Build history of the part. All positions in model axes, mm. A direction names the side the tool comes from. Give positions to 0.01 mm unless a question says otherwise; leave off trailing zeros. Write each loop counter-clockwise with the first axis right and the second up, starting at its lowest first coordinate (ties: lowest second). Pieces come first, ordered by that corner, then holes. Notation, with made-up numbers: (18, 35) -> (26, 35) arc R29 cw to (26, 55) -> close; hole circle Ø7 at (27, 81.5). An arc over 180 degrees is marked (long way). Put each result on its own line as item: value. Start each with the question number.
Item 1: Slice it at A-A, the plane x = 45.04. List the corners of the cut face in (y, z).
Item 2: Slice it at C-C, the plane z = -6.5. Give the number of separate pieces and of enclosed holes in the cut face, plus the area to 3 significant figures.
Item 3: Tool access for faces 4 (the flat face through (39, -45, -1.8)), 5 (the flat face through (39, -45, -8.3)), 6 (the flat face through (47.15, -32, -5)): list every direction of +Z, -Z, +X, -X, +Y, -Y with a clear straight run to the whole face (end or side of a thin tool).
Item 4: Flat gauge pins, fed straight in: pin 1 Ø4 at (x, z) = (39.5, -4.5) entering from -Y; pin 2 Ø3 at (x, z) = (48, -5.5) entering from +Y; pin 3 Ø1.3 at (y, z) = (-69, -5) entering from -X; pin 4 Ø1.5 at (y, z) = (-54.5, -1.5) entering from +X. Where does each tip first touch, or does it go through?
Item 5: Slice it at D-D, the plane x = 40. List the corners of the cut face in (y, z), plus the area to 3 significant figures.
Item 6: Slice it at B-B, the plane y = -31.5. List the corners of the cut face in (x, z), plus the area to 3 significant figures.
Item 7: Drill centre lines: line 1 along X through (y, z) = (-39.04, -4.25); line 2 along X through (y, z) = (-33, -6.75); line 3 along Y through (x, z) = (50.25, -6.5). Where is each one in solid material? Low to high.
Item 8: Two-plate mould, pull along X, no slides. Class faces 1 (the flat face through (52.05, -32, -5)), 2 (the flat face through (60.34, -60.4, -5.02)), 3 (the flat face through (60, -64, -2.925)): pulls with the +X half, pulls with the -X half, needs draft (parallel to the pull), parting line crosses it, or undercut.
```python
from build123d import *

# Parameters (mm, degrees)
SKETCH037_W             = 27.9
SKETCH037_H             = 15.9
SKETCH037_R             = 1.75
PAD025_DEPTH            = 9.9
SKETCH038_W             = 27.7
SKETCH038_H             = 4.25
REVOLUTION_ANGLE        = 10
SKETCH039_W             = 0.8
SKETCH039_H             = 6.5
PAD026_DEPTH            = 8.9
SKETCH040_W             = 0.8
SKETCH040_H             = 6.5
PAD027_DEPTH            = 3.5
SKETCH041_W             = 0.8
SKETCH041_H             = 6.5
PAD028_DEPTH            = 8.9
BODY007_PLACEMENT_ANGLE = 90


with BuildPart() as obj1:
    # Sketch037 → Pad025 (new body)
    with BuildSketch(Plane.XY):
        Rectangle(SKETCH037_W, SKETCH037_H)
        with Locations((10.96, 4.96)):
            Circle(SKETCH037_R, mode=Mode.SUBTRACT)
        with Locations((-10.96, -4.96)):
            Circle(SKETCH037_R, mode=Mode.SUBTRACT)
    extrude(amount=PAD025_DEPTH)

    # Sketch038 (on Face3 of Pad025) → Revolution (revolve)
    with BuildSketch(Plane.XZ.offset(7.95)):
        with Locations((10.8, 4.95)):
            Rectangle(SKETCH038_W, SKETCH038_H)
    revolve(axis=Axis((-3.15, -7.95, 7.075), (0, 0, -1)), revolution_arc=REVOLUTION_ANGLE)

    # Sketch039 (on Face2 of Revolution) → Pad026 (join)
    with BuildSketch(Plane(origin=(-13.95, 0, 0), x_dir=(0, -1, 0), z_dir=(-1, 0, 0))):
        with Locations((-2.45, 4.95)):
            Rectangle(SKETCH039_W, SKETCH039_H)
        with Locations((2.45, 4.95)):
            Rectangle(SKETCH039_W, SKETCH039_H)
    extrude(amount=PAD026_DEPTH)

    # Sketch040 (on Face1 of Pad026) → Pad027 (join)
    with BuildSketch(Plane(origin=(0, 7.95, 0), x_dir=(-1, 0, 0), z_dir=(0, 1, 0))):
        with Locations((1.55, 4.95)):
            Rectangle(SKETCH040_W, SKETCH040_H)
    extrude(amount=PAD027_DEPTH)

    # Sketch041 (on Face8 of Pad027) → Pad028 (join)
    with BuildSketch(Plane(origin=(-1.95, 0, 0), x_dir=(0, -1, 0), z_dir=(-1, 0, 0))):
        with Locations((-11.05, 4.95)):
            Rectangle(SKETCH041_W, SKETCH041_H)
    extrude(amount=PAD028_DEPTH)


with BuildPart() as obj1_1:
    # Body007 placement: moved
    add(obj1.part.moved(Location((50, 50, -10))).rotate(Axis((50, 50, -10), (0, 0, 1)), BODY007_PLACEMENT_ANGLE))


with BuildPart() as part_mirroring001:
    # Part__Mirroring001: instance of obj1
    add(obj1_1.part.mirror(Plane(origin=(0, 0, 0), x_dir=(1, 0, 0), z_dir=(0, 1, 0))))


solid = part_mirroring001.part
```
Values follow:
1. outline: (-63.95, -10) -> (-62.71, -10) -> (-62.71, -0.1) -> (-63.95, -0.1) -> close; (-59.21, -10) -> (-36.05, -10) -> (-36.05, -0.1) -> (-59.21, -0.1) -> close
2. separate pieces: 1
2. enclosed holes: 2
2. area: 516 mm2
3. face 4: +Z, -X, +Y, -Y
3. face 5: -Z, -X, +Y, -Y
3. face 6: +Z, -Z, -X, +Y
4. pin 1: y = -48.85
4. pin 2: y = -27.15
4. pin 3: x = 57.95
4. pin 4: x = 57.95
5. outline: (-48.85, -8.3) -> (-48.05, -8.3) -> (-48.05, -1.8) -> (-48.85, -1.8) -> close
5. area: 5.20 mm2
6. outline: (47.15, -8.3) -> (47.95, -8.3) -> (47.95, -1.8) -> (47.15, -1.8) -> close; (52.05, -8.3) -> (52.85, -8.3) -> (52.85, -1.8) -> (52.05, -1.8) -> close
6. area: 10.4 mm2
7. line 1: 42.05 to 53.21, 56.71 to 57.95
7. line 2: 47.15 to 47.95, 52.05 to 52.85
7. line 3: -63.95 to -36.05
8. face 1: undercut
8. face 2: pulls with the +X half
8. face 3: needs draft
